```python
from build123d import *

# Parameters (mm, degrees)
F1_DEPTH = 27.5
F2_R     = 3
F5_COUNT = 2
F6_R     = 0.5
F7_DEPTH = 3


with BuildPart() as f1:
    # F0 (on Right) → F1 (new body)
    with BuildSketch(Plane.YZ):
        Polygon((1.325824, 1.502603), (-1.502602, -1.325825), (-1.325825, -1.502602), (1.502601, 1.325827), align=None)
    extrude(amount=F1_DEPTH)

    # F2
    f2_edges = [f1.edges().sort_by_distance(p)[0] for p in [
        (27.5, 1.414212, 1.414215),
    ]]
    fillet(f2_edges, radius=F2_R)

    # F3 (on Front) → F4 (revolve)
    with BuildSketch(Plane.XZ):
        with BuildLine():
            Line((2.359792, -3.211392), (2.209123, 1.92127))
            ThreePointArc((2.209123, 1.92127), (1.53966, 3.441941), (0, 4.066495))
            Line((0, 4.066495), (0, -3.211392))
            Line((0, -3.211392), (2.359792, -3.211392))
        make_face()
    revolve(axis=Axis((0, 0, 0.427552), (0, 0, 1)))

    # F5: F1 ×2 about axis
    f5_axis = Axis((0, 0, -3.211392), (0, 0, 1))


with BuildPart() as f1_1:
    add(f1.part)
    for i in range(1, F5_COUNT):
        add(f1.part.rotate(f5_axis, i * 360 / F5_COUNT))

    # F6 (on face) → F7 (cut)
    with BuildSketch(Plane(origin=(0, 0, -3.211392), x_dir=(1, 0, 0), z_dir=(0, 0, -1))):
        Circle(F6_R)
    extrude(amount=-F7_DEPTH, mode=Mode.SUBTRACT)


solid = f1_1.part
```
Check sheet for the modelled part. Datum: model origin and axes. Units: mm. Give positions to 0.01 mm unless a question says otherwise; leave off trailing zeros. Order: outer loops, then holes, each group sorted by start corner. A loop starts at its lowest first (then second) coordinate and runs counter-clockwise, first axis right, second up. Notation, with made-up numbers: M -16.75,18 L 27.25,18 A23 ccw 27.25,53 Z; hole C 33,60.25 d2. An arc over 180 degrees is marked long. Answer in a Markdown table with one row per item. Add a question column.
Q1. Release check for a two-part mould opening along Z. For faces 1 (the flat face through (0, 0, -0.211)), 2 (the cylindrical face through (-0.108, 0.488, -1.732)), 3 (the flat face through (-14.443, 0.069, 0.108)), 4 (the conical face through (1.1, -2, -0.6)) record: released by +Z, released by -Z, zero draft, split by the parting line, or undercut.
Q2. Gauge pin test, flat ends, axial feed: pin 1 Ø4 at (x, z) = (-2, 2) entering from -Y; pin 2 Ø1 at (y, z) = (0, 2.5) entering from +X; pin 3 Ø1.5 at (x, y) = (21.5, -1) entering from +Z. Record the tip position at first contact, or that the pin passes through.
Q3. Thickness scan on L1, parallel to X at y = -0.4, z = 1; L2, parallel to X at y = 0, z = -2.2; L3, parallel to Y at x = 0, z = -2. Record the ranges inside material, lowest first.
Q4. Sectioned sample at A-A, the plane x = -22.5. Record the boundary of the cut face in (y, z).
Verdict:
| question | item | result |
|---|---|---|
| 1 | face 1 | released by -Z |
| 1 | face 2 | zero draft |
| 1 | face 3 | released by +Z |
| 1 | face 4 | undercut |
| 2 | pin 1 | y = -2.22 |
| 2 | pin 2 | x = 2.21 |
| 2 | pin 3 | z = -0.07 |
| 3 | L1 | -2.2 to 2.2 |
| 3 | L2 | -2.33 to -0.5, 0.5 to 2.33 |
| 3 | L3 | -2.32 to -0.5, 0.5 to 2.32 |
| 4 | outline | M -1.5,1.33 L 1.33,-1.5 L 1.5,-1.33 L -1.33,1.5 Z |
